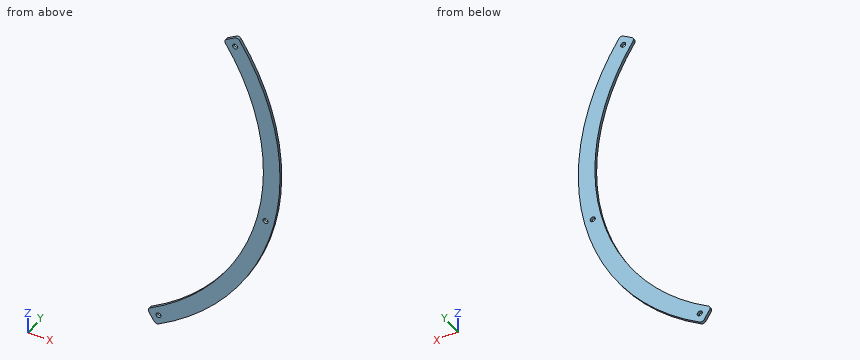
from build123d import *

# Parameters (mm, degrees)
BOSS_EXTRUDE1_DEPTH  = 1.75
MOUNTING_HOLES_REACH = 199.898
SKETCH2_R            = 1.55


with BuildPart() as part:
    # Sketch1 → Boss-Extrude1 (new body)
    with BuildSketch(Plane(origin=(0, 0, 0), x_dir=(1, 0, 0), z_dir=(0, 1, 0))):
        with BuildLine():
            Line((70.99149995, 123.045548212), (74.17169656, 128.134926657))
            ThreePointArc((74.17169656, 128.134926657), (75.398161995, 129.019168104), (76.893033195, 128.792319049))
            ThreePointArc((76.893033195, 128.792319049), (146.155509718, 33.742658152), (125.569837037, -82.050082429))
            ThreePointArc((125.569837037, -82.050082429), (124.325699782, -82.909281411), (122.835734015, -82.652177522))
            Line((122.835734015, -82.652177522), (117.74635557, -79.471980911))
            ThreePointArc((117.74635557, -79.471980911), (116.852809957, -78.205175291), (117.132867421, -76.680449723))
            ThreePointArc((117.132867421, -76.680449723), (136.41180907, 31.493147608), (71.663827182, 120.267601097))
            ThreePointArc((71.663827182, 120.267601097), (70.743717505, 121.515246248), (70.99149995, 123.045548212))
        make_face()
    extrude(amount=BOSS_EXTRUDE1_DEPTH)

    # Sketch2 → Mounting_Holes (cut, up to next)
    with BuildSketch(Plane(origin=(0, 1.75, 0), x_dir=(1, 0, 0), z_dir=(0, 1, 0)), mode=Mode.PRIVATE) as mounting_holes_sk1:
        with Locations(Location((122.966973943, -76.838293314, 0), (0, 0, 270))):
            Circle(SKETCH2_R)
    mounting_holes_tool1 = extrude(mounting_holes_sk1.sketch, amount=-MOUNTING_HOLES_REACH, mode=Mode.PRIVATE) & part.part
    # Sketch2 → Mounting_Holes (cut, up to next)
    with BuildSketch(Plane(origin=(0, 1.75, 0), x_dir=(1, 0, 0), z_dir=(0, 1, 0)), mode=Mode.PRIVATE) as mounting_holes_sk2:
        with Locations(Location((141.283659394, 32.61790288, 0), (0, 0, 270))):
            Circle(SKETCH2_R)
    mounting_holes_tool2 = extrude(mounting_holes_sk2.sketch, amount=-MOUNTING_HOLES_REACH, mode=Mode.PRIVATE) & part.part
    # Sketch2 → Mounting_Holes (cut, up to next)
    with BuildSketch(Plane(origin=(0, 1.75, 0), x_dir=(1, 0, 0), z_dir=(0, 1, 0)), mode=Mode.PRIVATE) as mounting_holes_sk3:
        with Locations(Location((76.838293314, 122.966973943, 0), (0, 0, 270))):
            Circle(SKETCH2_R)
    mounting_holes_tool3 = extrude(mounting_holes_sk3.sketch, amount=-MOUNTING_HOLES_REACH, mode=Mode.PRIVATE) & part.part
    add(mounting_holes_tool1.solids().sort_by_distance((122.966974, 1.75, 76.838293))[0], mode=Mode.SUBTRACT)
    add(mounting_holes_tool2.solids().sort_by_distance((141.283659, 1.75, -32.617903))[0], mode=Mode.SUBTRACT)
    add(mounting_holes_tool3.solids().sort_by_distance((76.838293, 1.75, -122.966974))[0], mode=Mode.SUBTRACT)


solid = part.part
The listing builds one solid part. Answer for the finished solid, in the listing's coordinates (mm). Give positions to 0.01 mm unless a question says otherwise; leave off trailing zeros. Order: outer loops, then holes, each group sorted by start corner. A loop starts at its lowest first (then second) coordinate and runs counter-clockwise, first axis right, second up. Notation, with made-up numbers: (-14.5, 25) -> (38.5, 25) arc R29 cw to (38.5, 53) -> close; hole circle Ø4 at (48, 56.5). An arc over 180 degrees is marked (long way). Put each result on its own line as item: value.
Item 1: Straight lines are drawn through the part: line 1 (Z direction, x = 123, y = 0.1); line 2 (Z direction, x = 126, y = 1.6); line 3 (Z direction, x = 119.5, y = 1.05). For each, find the intervals that lie inside material, in ascending order.
Established:
line 1: z = -85.85 to -66.87, 66.87 to 75.29, 78.39 to 82.74
line 2: z = -81.39 to -61.02, 61.02 to 81.39
line 3: z = -90.66 to -72.94, 72.94 to 80.57
Item 2: A cutting plane is placed at A-A on y = 1.35. Give the vertices of the cut face in (x, z).
Established:
outline: (70.99, -123.05) -> (74.17, -128.13) arc R2 ccw to (76.89, -128.79) arc R150 ccw to (125.57, 82.05) arc R2 ccw to (122.84, 82.65) -> (117.75, 79.47) arc R2 ccw to (117.13, 76.68) arc R140 cw to (71.66, -120.27) arc R2 ccw to start; hole circle Ø3.1 at (76.84, -122.97); hole circle Ø3.1 at (122.97, 76.84); hole circle Ø3.1 at (141.28, -32.62)
Item 3: Given P1, Ø1, axis at y = 0.5, z = 36.5, coming from the -X side; P2, Ø1, axis at y = 0.5, z = -16.5, coming from the -X side, each flat-ended and moving along its own axis, determine where each tip first touches the part or whether it passes through.
Established:
P1: stops at x = 135.02
P2: stops at x = 138.96
Item 4: A cutting plane is placed at C-C on z = -115. Give the vertices of the cut face in (x, y), plus the area to 3 significant figures.
Established:
outline: (79.84, 0) -> (96.31, 0) -> (96.31, 1.75) -> (79.84, 1.75) -> close
area: 28.8 mm^2
Item 5: A cutting plane is placed at B-B on x = 131.5. Give the vertices of the cut face in (y, z), plus the area to 3 significant figures.
Established:
outline: (0, -72.16) -> (1.75, -72.16) -> (1.75, -48.04) -> (0, -48.04) -> close; (0, 48.04) -> (1.75, 48.04) -> (1.75, 72.16) -> (0, 72.16) -> close
area: 84.4 mm^2
Item 6: A cutting plane is placed at D-D on x = 84.5. Give the vertices of the cut face in (y, z), plus the area to 3 significant figures.
Established:
outline: (0, -123.93) -> (1.75, -123.93) -> (1.75, -111.62) -> (0, -111.62) -> close
area: 21.5 mm^2
